Check sheet for the modelled part. Datum: model origin and axes. Units: mm. Coordinates: 2 decimals unless noted, no trailing zeros. Order: outer loops, then holes, each group sorted by start corner. A loop starts at its lowest first (then second) coordinate and runs counter-clockwise, first axis right, second up.
1. Gauge pin test, flat ends, axial feed: pin 1 Ø0.9 at (x, y) = (-0.5, -27.5) entering from +Z; pin 2 Ø0.9 at (x, y) = (-0.5, 34.5) entering from -Z; pin 3 Ø1.6 at (x, y) = (0, 33.5) entering from +Z. Record the tip position at first contact, or that the pin passes through.
2. Cross-section at D-D (y = 23). Enter the section's corners in (x, z).
3. Cross-section at A-A (z = 37). Enter the section's corners in (x, y).
4. Cross-section at B-B (y = -16.1). Enter the section's corners in (x, z).
5. Thickness scan on line 1 (Y direction, x = -0.25, z = -4.6); line 2 (Z direction, x = 0.25, y = -33.5); line 3 (Y direction, x = -0.85, z = -25.2). Record the ranges inside material, lowest first.
6. Cross-section at C-C (x = 0.25). Count the separate pieces of the cut face and the enclosed holes in it, then the cut area to 3 significant figures.
```python
from build123d import *

# Parameters (mm, degrees)
CROQUIS1_W               = 108
CROQUIS1_H               = 71
SALIENTE_EXTRUIR1_DEPTH  = 1.5
CROQUIS2_W               = 12
CROQUIS2_H               = 3
CROQUIS2_W_2             = 8
CORTAR_EXTRUIR1_DEPTH    = 3
CROQUIS6_W               = 3
CROQUIS6_H               = 14
CROQUIS6_H_2             = 8
CORTAR_EXTRUIR3_DEPTH    = 3
CROQUIS8_W               = 8
CROQUIS8_H               = 3
SALIENTE_EXTRUIR2_DEPTH  = 3
REDONDEO2_R              = 4
CROQUIS9_R               = 1.5
CORTAR_EXTRUIR5_DEPTH    = 3
REDONDEO2_OF_SIMETR_A1_R = 4
CROQUIS12_W              = 12.481361742
CROQUIS12_H              = 10.4
CROQUIS12_W_2            = 12.356019523
CORTAR_EXTRUIR7_DEPTH    = 10
CROQUIS10_R              = 4.6
CROQUIS10_R_2            = 3.5
CROQUIS10_R_3            = 2
CROQUIS10_W              = 4.5
CROQUIS10_H              = 7
CORTAR_EXTRUIR6_DEPTH    = 10
CROQUIS14_R              = 5
CROQUIS14_R_2            = 0.007419035
CORTAR_EXTRUIR9_DEPTH    = 10


with BuildPart() as part:
    # Croquis1 → Saliente-Extruir1 (new, symmetric)
    with BuildSketch(Plane(origin=(0, 0, 0), x_dir=(0, 0, -1), z_dir=(1, 0, 0))):
        Rectangle(CROQUIS1_W, CROQUIS1_H)
    extrude(amount=SALIENTE_EXTRUIR1_DEPTH, both=True)

    # Croquis2 → Cortar-Extruir1 (cut)
    with BuildSketch(Plane.ZY.offset(1.5)):
        with Locations((-48, -34)):
            Rectangle(CROQUIS2_W, CROQUIS2_H)
        with Locations((-8, -34)):
            Rectangle(CROQUIS2_W_2, CROQUIS2_H)
        with Locations((48, 34)):
            Rectangle(CROQUIS2_W, CROQUIS2_H)
        with Locations((24, 34)):
            Rectangle(CROQUIS2_W_2, CROQUIS2_H)
        with Locations((8, 34)):
            Rectangle(CROQUIS2_W_2, CROQUIS2_H)
        with Locations((-8, 34)):
            Rectangle(CROQUIS2_W_2, CROQUIS2_H)
        with Locations((-24, 34)):
            Rectangle(CROQUIS2_W_2, CROQUIS2_H)
        with Locations((-48, 34)):
            Rectangle(CROQUIS2_W, CROQUIS2_H)
        with Locations((8, -34)):
            Rectangle(CROQUIS2_W_2, CROQUIS2_H)
        with Locations((24, -34)):
            Rectangle(CROQUIS2_W_2, CROQUIS2_H)
    extrude(amount=-CORTAR_EXTRUIR1_DEPTH, mode=Mode.SUBTRACT)

    # Croquis6 → Cortar-Extruir3 (cut)
    with BuildSketch(Plane.ZY.offset(1.5)):
        with Locations((52.5, -28.5)):
            Rectangle(CROQUIS6_W, CROQUIS6_H)
        with Locations((52.5, -6.5)):
            Rectangle(CROQUIS6_W, CROQUIS6_H_2)
        with Locations((52.5, 6.5)):
            Rectangle(CROQUIS6_W, CROQUIS6_H_2)
        with Locations((52.5, 28.5)):
            Rectangle(CROQUIS6_W, CROQUIS6_H)
    extrude(amount=-CORTAR_EXTRUIR3_DEPTH, mode=Mode.SUBTRACT)

    # Croquis8 → Saliente-Extruir2 (add)
    with BuildSketch(Plane.ZY.offset(1.5)):
        with Locations((16, 37)):
            Rectangle(CROQUIS8_W, CROQUIS8_H)
    saliente_extruir2 = extrude(amount=-SALIENTE_EXTRUIR2_DEPTH)

    # Redondeo2
    redondeo2_edges = [part.edges().sort_by_distance(p)[0] for p in [
        (0, 38.5, 20),
        (0, 38.5, 12),
    ]]
    fillet(redondeo2_edges, radius=REDONDEO2_R - 0.0001)  # a hair under: the kernel refuses the full size

    # Croquis9 → Cortar-Extruir5 (cut)
    with BuildSketch(Plane.ZY.offset(1.5)):
        with Locations((16, 33.5)):
            Circle(CROQUIS9_R)
    cortar_extruir5 = extrude(amount=-CORTAR_EXTRUIR5_DEPTH, mode=Mode.SUBTRACT)

    # Simetría1: Saliente-Extruir2, Cortar-Extruir5 across plane
    add(saliente_extruir2.mirror(Plane.ZX))
    add(cortar_extruir5.mirror(Plane.ZX), mode=Mode.SUBTRACT)

    # Redondeo2 of Simetría1
    redondeo2_of_simetr_a1_edges = [part.edges().sort_by_distance(p)[0] for p in [
        (0, -38.5, 20),
        (0, -38.5, 12),
    ]]
    fillet(redondeo2_of_simetr_a1_edges, radius=REDONDEO2_OF_SIMETR_A1_R - 0.0001)  # a hair under: the kernel refuses the full size

    # Croquis12 → Cortar-Extruir7 (cut)
    with BuildSketch(Plane.ZY.offset(1.5)):
        with Locations((36.9, -27.305454422)):
            Rectangle(CROQUIS12_W, CROQUIS12_H)
        with Locations((-32.051890368, -27.305454422)):
            Rectangle(CROQUIS12_W_2, CROQUIS12_H)
    extrude(amount=-CORTAR_EXTRUIR7_DEPTH, mode=Mode.SUBTRACT)

    # Croquis10 → Cortar-Extruir6 (cut)
    with BuildSketch(Plane.ZY.offset(1.5)):
        with Locations((-25.2, -16.1)):
            Circle(CROQUIS10_R)
        with Locations((-14.4, -16.1)):
            Circle(CROQUIS10_R_2)
        with Locations((-4.6, -24.85)):
            Circle(CROQUIS10_R_3)
        with Locations((6.85, -16.1)):
            Rectangle(CROQUIS10_W, CROQUIS10_H)
        with Locations((-4.6, -7.35)):
            Circle(CROQUIS10_R_3)
    extrude(amount=-CORTAR_EXTRUIR6_DEPTH, mode=Mode.SUBTRACT)

    # Croquis14 → Cortar-Extruir9 (cut)
    with BuildSketch(Plane(origin=(1.5, 0, 0), x_dir=(0, 0, -1), z_dir=(1, 0, 0))):
        with Locations((25.2, -16.1)):
            Circle(CROQUIS14_R)
        with Locations((21.161787618, -13.912617849)):
            Circle(CROQUIS14_R_2, mode=Mode.SUBTRACT)
    extrude(amount=-CORTAR_EXTRUIR9_DEPTH, mode=Mode.SUBTRACT)


solid = part.part
```
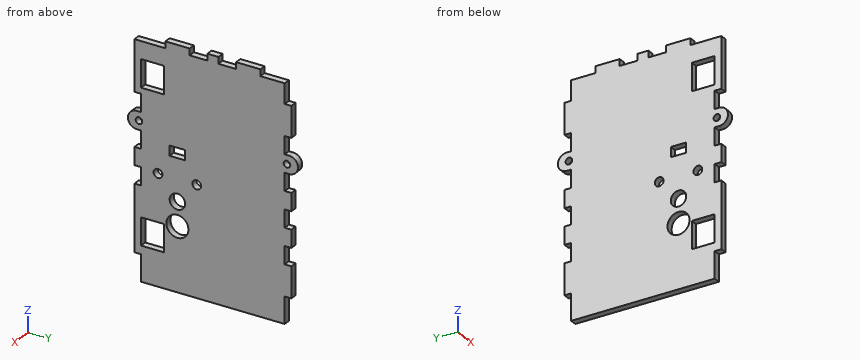
Data:
1. pin 1: stops at z = 51
1. pin 2: stops at z = -42
1. pin 3: stops at z = 42
2. outline: (-1.5, -54) - (1.5, -54) - (1.5, 51) - (-1.5, 51) - close
3. outline: (-1.5, -35.5) - (1.5, -35.5) - (1.5, -32.51) - (-1.5, -32.51) - close; (-1.5, -22.11) - (1.5, -22.11) - (1.5, 35.5) - (-1.5, 35.5) - close
4. outline: (-1.5, -54) - (1.5, -54) - (1.5, -30.2) - (-1.5, -30.2) - close; (-1.5, -20.2) - (1.5, -20.2) - (1.5, -17.9) - (-1.5, -17.9) - close; (-1.5, -10.9) - (1.5, -10.9) - (1.5, 4.6) - (-1.5, 4.6) - close; (-1.5, 9.1) - (1.5, 9.1) - (1.5, 54) - (-1.5, 54) - close
5. line 1: y = -32.5 to -26.85, -22.85 to -9.35, -5.35 to 32.5
5. line 2: z = -42 to -12, -4 to 4, 12 to 14.5, 17.5 to 20, 28 to 51
5. line 3: y = -35.5 to -21.1, -11.1 to 32.5
6. separate pieces: 1
6. enclosed holes: 9
6. area: 6,860 mm2
